Here's how the part is built. I have some questions about the finished solid (model axes, mm). A direction names the side the tool comes from. Give positions to 0.01 mm unless a question says otherwise; leave off trailing zeros. Loops run counter-clockwise (first coordinate to the right, second up) from the corner with the lowest first, then second, coordinate; pieces in that order, holes last. Notation, with made-up numbers: (-19.5, 69) - (19.5, 69) arc R12 ccw to (19.5, 87) - close; hole circle Ø9 at (64.5, 21). An arc over 180 degrees is marked (long way). Use one line per item in the form item = value.
from build123d import *

# Parameters (mm, degrees)
F1_DEPTH = 70
F3_DEPTH = 63.55
F4_DEPTH = 6.45
F6_D     = 8.6106
F6_DEPTH = 20
F6_TIP   = 2.5868852231


with BuildPart() as f1:
    # F0 (on Top) → F1 (new body)
    with BuildSketch(Plane.XY):
        with BuildLine():
            Line((0, -39.35), (25.55, -39.35))
            Line((25.55, -39.35), (25.55, 13.8))
            Line((25.55, 13.8), (19.1, 13.8))
            ThreePointArc((19.1, 13.8), (13.5057395207, 0.2942604793), (0, -5.3))
            Line((0, -5.3), (0, -39.35))
        make_face()
        with BuildLine():
            Line((-25.55, -39.35), (0, -39.35))
            Line((0, -39.35), (0, -5.3))
            ThreePointArc((0, -5.3), (-13.5057395207, 0.2942604793), (-19.1, 13.8))
            Line((-19.1, 13.8), (-25.55, 13.8))
            Line((-25.55, 13.8), (-25.55, -39.35))
        make_face()
        with BuildLine():
            Line((19.1, 13.8), (25.55, 13.8))
            Line((25.55, 13.8), (25.55, 39.35))
            Line((25.55, 39.35), (0, 39.35))
            Line((0, 39.35), (0, 32.9))
            ThreePointArc((0, 32.9), (13.5057395207, 27.3057395207), (19.1, 13.8))
        make_face()
        with BuildLine():
            Line((-25.55, 39.35), (-25.55, 13.8))
            Line((-25.55, 13.8), (-19.1, 13.8))
            ThreePointArc((-19.1, 13.8), (-13.5057395207, 27.3057395207), (0, 32.9))
            Line((0, 32.9), (0, 39.35))
            Line((0, 39.35), (-25.55, 39.35))
        make_face()
        with BuildLine():
            Line((0, 13.8), (19.1, 13.8))
            ThreePointArc((19.1, 13.8), (13.5057395207, 27.3057395207), (0, 32.9))
            Line((0, 32.9), (0, 13.8))
        make_face()
        with BuildLine():
            Line((0, 13.8), (0, -5.3))
            ThreePointArc((0, -5.3), (13.5057395207, 0.2942604793), (19.1, 13.8))
            Line((19.1, 13.8), (0, 13.8))
        make_face()
        with BuildLine():
            ThreePointArc((-19.1, 13.8), (-13.5057395207, 0.2942604793), (0, -5.3))
            Line((0, -5.3), (0, 13.8))
            Line((0, 13.8), (-19.1, 13.8))
        make_face()
        with BuildLine():
            Line((-19.1, 13.8), (0, 13.8))
            Line((0, 13.8), (0, 32.9))
            ThreePointArc((0, 32.9), (-13.5057395207, 27.3057395207), (-19.1, 13.8))
        make_face()
    extrude(amount=F1_DEPTH)

    # F0 (on Top) → F3 (cut)
    with BuildSketch(Plane.XY):
        with BuildLine():
            Line((-19.1, 13.8), (0, 13.8))
            Line((0, 13.8), (0, 32.9))
            ThreePointArc((0, 32.9), (-13.5057395207, 27.3057395207), (-19.1, 13.8))
        make_face()
        with BuildLine():
            Line((0, 13.8), (19.1, 13.8))
            ThreePointArc((19.1, 13.8), (13.5057395207, 27.3057395207), (0, 32.9))
            Line((0, 32.9), (0, 13.8))
        make_face()
        with BuildLine():
            Line((0, 13.8), (0, -5.3))
            ThreePointArc((0, -5.3), (13.5057395207, 0.2942604793), (19.1, 13.8))
            Line((19.1, 13.8), (0, 13.8))
        make_face()
        with BuildLine():
            ThreePointArc((-19.1, 13.8), (-13.5057395207, 0.2942604793), (0, -5.3))
            Line((0, -5.3), (0, 13.8))
            Line((0, 13.8), (-19.1, 13.8))
        make_face()
    extrude(amount=F3_DEPTH, mode=Mode.SUBTRACT)

    # F2 (on face) → F4 (cut)
    with BuildSketch(Plane.XY.offset(70)):
        with BuildLine():
            Line((0, 5.25), (0, 13.8))
            Line((0, 13.8), (-8.55, 13.8))
            ThreePointArc((-8.55, 13.8), (-6.0457629791, 7.7542370209), (0, 5.25))
        make_face()
        with BuildLine():
            Line((8.55, 13.8), (0, 13.8))
            Line((0, 13.8), (0, 5.25))
            ThreePointArc((0, 5.25), (6.0457629791, 7.7542370209), (8.55, 13.8))
        make_face()
        with BuildLine():
            ThreePointArc((8.55, 13.8), (6.0457629791, 19.8457629791), (0, 22.35))
            Line((0, 22.35), (0, 13.8))
            Line((0, 13.8), (8.55, 13.8))
        make_face()
        with BuildLine():
            Line((0, 13.8), (0, 22.35))
            ThreePointArc((0, 22.35), (-6.0457629791, 19.8457629791), (-8.55, 13.8))
            Line((-8.55, 13.8), (0, 13.8))
        make_face()
    extrude(amount=-F4_DEPTH, mode=Mode.SUBTRACT)

    # F6
    with Locations(Plane.XZ.offset(39.35)):
        with Locations((-15, 55), (15, 55), (15, 45), (-15, 45)):
            Hole(F6_D / 2, depth=F6_DEPTH)
            with Locations((0, 0, -(F6_DEPTH + F6_TIP / 2))):  # 118° drill point
                Cone(0, F6_D / 2, F6_TIP, mode=Mode.SUBTRACT)


solid = f1.part
(1) If we section it at A-A (z = 7): List the corners of the cut face in (x, y) for me, plus the area to 3 significant figures.
Geometry says:
outline = (-25.55, -39.35) - (25.55, -39.35) - (25.55, 39.35) - (-25.55, 39.35) - close; hole circle Ø38.2 at (0, 13.8)
area = 2,880 mm²
(2) Thinking about a two-plate mould opening in Z: for faces 1 (the flat face through (0, 39.35, 35)), 2 (the flat face through (4, 6, 63.55)), 3 (the cylindrical face through (-17.315, -29.21, 48.63)), which applies, pulls with the +Z half, pulls with the -Z half, needs draft (parallel to the pull), parting line crosses it, or undercut?
Geometry says:
face_1 = needs draft
face_2 = pulls with the -Z half
face_3 = undercut
(3) For P1, Ø4, axis at x = -7.5, y = 27.5, coming from the -Z side; P2, Ø6, axis at x = 15.5, y = 24, coming from the -Z side, each with a flat end and sliding along its axis, tell me the tip position at first contact or that it passes through.
Geometry says:
P1 = 63.55
P2 = 0
(4) If we section it at B-B (y = 16.5): List the corners of the cut face in (x, z) for me, plus the area to 3 significant figures.
Geometry says:
outline = (-25.55, 0) - (-18.91, 0) - (-18.91, 63.55) - (-8.11, 63.55) - (-8.11, 70) - (-25.55, 70) - close; (8.11, 63.55) - (18.91, 63.55) - (18.91, 0) - (25.55, 0) - (25.55, 70) - (8.11, 70) - close
area = 1,070 mm²
(5) If we section it at C-C (x = 2): List the corners of the cut face in (y, z) for me (3 decimals), plus the area to 3 significant figures.
Geometry says:
outline = (-39.35, 0) - (-5.195, 0) - (-5.195, 63.55) - (5.487, 63.55) - (5.487, 70) - (-39.35, 70) - close; (22.113, 63.55) - (32.795, 63.55) - (32.795, 0) - (39.35, 0) - (39.35, 70) - (22.113, 70) - close
area = 2,990 mm²
(6) For faces 4 (the cylindrical face through (15.56, -29.21, 59.27)), 5 (the flat face through (0, -39.35, 35)), which set-ups out of +Z, -Z, +X, -X, +Y, -Y let a thin tool reach every point of the face, with its end or its side?
Geometry says:
face_4 = -Y
face_5 = +Z, -Z, +X, -X, -Y
(7) If I drill on probe 1 along Z at (x, y) = (15, -27); probe 2 along X at (y, z) = (-35, 45); probe 3 along X at (y, z) = (0.5, 59), over which ranges is the centre line in solid material (lowest first)?
Geometry says:
probe_1 = 0 to 40.69, 49.31 to 50.69, 59.31 to 70
probe_2 = -25.55 to -19.31, -10.69 to 10.69, 19.31 to 25.55
probe_3 = -25.55 to -13.71, 13.71 to 25.55
